Autodesk Inventor part; units mm, degrees
ref_plane "YZ Plane" through (0, 0, 0) normal (1, 0, 0) x (0, 1, 0)
ref_plane "XZ Plane" through (0, 0, 0) normal (0, 1, 0) x (-1, 0, 0)
ref_plane "XY Plane" through (0, 0, 0) normal (0, 0, 1) x (1, 0, 0)
sketch "Sketch1" plane through (0, 0, 0) normal (0, 0, 1) x (1, 0, 0)
  line L0 (5, 0) -> (336, 0)
  line L1 (341, 5) -> (341, 96)
  line L2 (336, 101) -> (5, 101)
  line L3 (0, 96) -> (0, 5)
  arc A0 (5, 101) -> (0, 96) centre (5, 96) ccw
  arc A1 (0, 5) -> (5, 0) centre (5, 5) ccw
  arc A2 (341, 96) -> (336, 101) centre (336, 96) ccw
  arc A3 (336, 0) -> (341, 5) centre (336, 5) ccw
  line L4 (5, 101.2) -> (336, 101.2)
  arc A4 (341.2, 96) -> (336, 101.2) centre (336, 96) ccw
  line L5 (341.2, 96) -> (341.2, 5)
  arc A5 (336, -0.2) -> (341.2, 5) centre (336, 5) ccw
  line L6 (336, -0.2) -> (5, -0.2)
  arc A6 (-0.2, 5) -> (5, -0.2) centre (5, 5) ccw
  line L7 (-0.2, 5) -> (-0.2, 96)
  arc A7 (5, 101.2) -> (-0.2, 96) centre (5, 96) ccw
  line L8 (5, 104) -> (336, 104)
  arc A8 (344, 96) -> (336, 104) centre (336, 96) ccw
  line L9 (344, 96) -> (344, 5)
  arc A9 (336, -3) -> (344, 5) centre (336, 5) ccw
  line L10 (336, -3) -> (5, -3)
  arc A10 (-3, 5) -> (5, -3) centre (5, 5) ccw
  line L11 (-3, 5) -> (-3, 96)
  arc A11 (5, 104) -> (-3, 96) centre (5, 96) ccw
  point P0 (0, 0)
  point P1 (341, 101)
  point P2 (0, 101)
  dimension "d0" = 341
  dimension "d1" = 101
  dimension "d2" = 5
  dimension "d3" = 0.2
  dimension "d4" = 3
extrude "Extrusion1" add sketch "Sketch1" along normal blind 2 contours A1 L3 A0 L2 A2 L1 A3 L0 | L4 A4 L5 A5 L6 A6 L7 A7 | L8 A8 L9 A9 L10 A10 L11 A11
sketch "Sketch2" plane through (0, 0, 2) normal (0, 0, 1) x (1, 0, 0)
  line L0 (5, 104) -> (336, 104)
  line L1 (344, 96) -> (344, 5)
  line L2 (336, -3) -> (5, -3)
  line L3 (-3, 5) -> (-3, 96)
  line L4 (344, 5) -> (344, 96)
  line L5 (5, -3) -> (336, -3)
  arc A0 (5, 104) -> (-3, 96) centre (5, 96) ccw
  arc A1 (-3, 5) -> (5, -3) centre (5, 5) ccw
  arc A2 (336, -3) -> (344, 5) centre (336, 5) ccw
  arc A3 (344, 96) -> (336, 104) centre (336, 96) ccw
  line L6 (336, 101.2) -> (5, 101.2)
  arc A4 (5, 101.2) -> (-0.2, 96) centre (5, 96) ccw
  line L7 (-0.2, 96) -> (-0.2, 5)
  arc A5 (-0.2, 5) -> (5, -0.2) centre (5, 5) ccw
  line L8 (5, -0.2) -> (336, -0.2)
  arc A6 (336, -0.2) -> (341.2, 5) centre (336, 5) ccw
  line L9 (341.2, 5) -> (341.2, 96)
  arc A7 (341.2, 96) -> (336, 101.2) centre (336, 96) ccw
  circle A8 centre (5, 96) radius 2.5
  line L10 (9, 92) -> (332, 92)
  line L11 (332, 92) -> (332, 9)
  line L12 (332, 9) -> (9, 9)
  line L13 (9, 9) -> (9, 92)
  line L14 (-0.2, 89.2) -> (8, 89.2)
  line L15 (8, 89.2) -> (8, 93)
  line L16 (8, 93) -> (11.8, 93)
  line L17 (11.8, 93) -> (11.8, 101.2)
  line L18 (9, 9) -> (332, 92)
  line L19 (170.5, 64.427) -> (170.5, 38.8649)
  line L20 (118.7328, 50.5) -> (212.1169, 50.5)
  circle A9 centre (336, 96) radius 2.5
  line L21 (341.2, 89.2) -> (333, 89.2)
  line L22 (333, 89.2) -> (333, 93)
  line L23 (333, 93) -> (329.2, 93)
  line L24 (329.2, 93) -> (329.2, 101.2)
  circle A10 centre (5, 5) radius 2.5
  line L25 (-0.2, 11.8) -> (8, 11.8)
  line L26 (8, 11.8) -> (8, 8)
  line L27 (8, 8) -> (11.8, 8)
  line L28 (11.8, 8) -> (11.8, -0.2)
  line L29 (329.2, 8) -> (329.2, -0.2)
  line L30 (333, 8) -> (329.2, 8)
  line L31 (333, 11.8) -> (333, 8)
  line L32 (341.2, 11.8) -> (333, 11.8)
  circle A11 centre (336, 5) radius 2.5
  point P0 (0, 0)
  dimension "d7" = 0
  dimension "d8" = 0
  dimension "d9" = 8
  dimension "d10" = 2.8
  dimension "d11" = 5
  dimension "d12" = 5.2
  dimension "d13" = 5.2
  dimension "d19" = 9.2
  dimension "d20" = 9.2
  dimension "d21" = 9.2
  dimension "d22" = 9.2
  dimension "d23" = 1
  dimension "d24" = 1
  dimension "d25" = 12
  dimension "d26" = 12
extrude "Extrusion2" add sketch "Sketch2" along normal blind 30 contours L0 A3 L1 A2 L2 A1 L3 A0 | A7 L9 L21 L22 L23 L24 L6 | L17 L16 L15 L14 L7 A4 L6 | L9 A6 L8 L29 L30 L31 L32 | L25 L26 L27 L28 L8 A5 L7
sketch "Sketch3" plane through (0, 0, 32) normal (0, 0, 1) x (1, 0, 0)
  line L0 (5, 104) -> (336, 104)
  line L1 (344, 96) -> (344, 5)
  line L2 (336, -3) -> (5, -3)
  line L3 (-3, 5) -> (-3, 96)
  arc A0 (5, 104) -> (-3, 96) centre (5, 96) ccw
  arc A1 (-3, 5) -> (5, -3) centre (5, 5) ccw
  arc A2 (336, -3) -> (344, 5) centre (336, 5) ccw
  arc A3 (344, 96) -> (336, 104) centre (336, 96) ccw
  line L4 (336, 101.2) -> (5, 101.2)
  arc A4 (5, 101.2) -> (-0.2, 96) centre (5, 96) ccw
  line L5 (-0.2, 96) -> (-0.2, 5)
  arc A5 (-0.2, 5) -> (5, -0.2) centre (5, 5) ccw
  line L6 (5, -0.2) -> (336, -0.2)
  arc A6 (336, -0.2) -> (341.2, 5) centre (336, 5) ccw
  line L7 (341.2, 5) -> (341.2, 96)
  arc A7 (341.2, 96) -> (336, 101.2) centre (336, 96) ccw
  point P0 (0, 0)
  dimension "d29" = 8
  dimension "d30" = 2.8
extrude "Extrusion3" add sketch "Sketch3" along normal blind 7
sketch "Sketch4" plane through (0, 0, 2) normal (0, 0, 1) x (1, 0, 0)
  line L0 (336, -0.2) -> (5, -0.2)
  line L1 (157.75, -0.2) -> (183.25, -0.2)
  line L2 (183.25, -0.2) -> (183.25, 48.2)
  line L3 (183.25, 48.2) -> (157.75, 48.2)
  line L4 (157.75, 48.2) -> (157.75, -0.2)
  line L5 (-0.2, 5) -> (-0.2, 96)
  circle A0 centre (160.25, 45.7) radius 2.3
  circle A1 centre (180.75, 45.7) radius 2.3
  circle A2 centre (160.25, 2.3) radius 2.3
  circle A3 centre (180.75, 2.3) radius 2.3
  point P0 (0, 0)
  dimension "d33" = 25.5
  dimension "d34" = 48.4
  dimension "d35" = 157.95
  dimension "d36" = 4.6
  dimension "d37" = 4.6
  dimension "d38" = 4.6
  dimension "d39" = 4.6
  dimension "d40" = 2.5
  dimension "d41" = 2.5
  dimension "d42" = 2.5
  dimension "d43" = 2.5
  dimension "d44" = 2.5
  dimension "d45" = 2.5
  dimension "d46" = 2.5
  dimension "d47" = 2.5
extrude "Extrusion4" add sketch "Sketch4" along normal blind 4 contours A0 | A1 | A2 | A3
sketch "Sketch5" plane through (160.25, 2.3, 6) normal (0, 0, 1) x (1, 0, 0)
  circle A0 centre (0, 43.4) radius 2.3
  circle A1 centre (0, 43.4) radius 1.5
  circle A2 centre (20.5, 43.4) radius 2.3
  circle A3 centre (20.5, 43.4) radius 1.5
  circle A4 centre (0, 0) radius 2.3
  circle A5 centre (0, 0) radius 1.5
  circle A6 centre (20.5, 0) radius 2.3
  circle A7 centre (20.5, 0) radius 1.5
  point P0 (-160.25, -2.3)
  dimension "d50" = 3
  dimension "d51" = 3
  dimension "d52" = 3
  dimension "d53" = 3
extrude "Extrusion5" add sketch "Sketch5" along normal blind 3 contours A1 | A3
chamfer "Chamfer1" distance 1 angle 45 2 edges at (158.75, 45.7, 9) (179.25, 45.7, 9)
sketch "Sketch6" plane through (5, -3, 0) normal (0, -1, 0) x (1, 0, 0)
  line L0 (161.3, 2.8) -> (169.7, 2.8)
  line L1 (169.7, 2.8) -> (169.7, 6.2)
  line L2 (169.7, 6.2) -> (161.3, 6.2)
  line L3 (161.3, 6.2) -> (161.3, 2.8)
  line L4 (6.8, 2) -> (324.2, 2)
  line L5 (0, 0) -> (0, 39)
  point P0 (-5, 0)
  dimension "d59" = 8.4
  dimension "d60" = 3.4
  dimension "d61" = 4.2
  dimension "d62" = 161.3
extrude "Extrusion6" cut sketch "Sketch6" against normal blind 3
sketch "Sketch7" plane through (0, 0, 2) normal (0, 0, 1) x (1, 0, 0)
  line L0 (99.8, 7.8) -> (107.8, 7.8)
  line L1 (107.8, 7.8) -> (107.8, 10.8)
  line L2 (107.8, 10.8) -> (99.8, 10.8)
  line L3 (99.8, 10.8) -> (99.8, 7.8)
  line L4 (336, -0.2) -> (5, -0.2)
  line L5 (-0.2, 5) -> (-0.2, 96)
  point P0 (0, 0)
  dimension "d65" = 8
  dimension "d66" = 3
  dimension "d67" = 8
  dimension "d68" = 100
extrude "Extrusion7" cut sketch "Sketch7" against normal blind 3
sketch "Sketch8" plane through (0, 0, 2) normal (0, 0, 1) x (1, 0, 0)
  line L0 (11.8, -0.2) -> (329.2, -0.2)
  line L1 (95.8, -0.2) -> (111.8, -0.2)
  line L2 (111.8, -0.2) -> (111.8, 5.95)
  line L3 (111.8, 5.95) -> (95.8, 5.95)
  line L4 (95.8, 5.95) -> (95.8, -0.2)
  line L5 (107.8, 7.8) -> (99.8, 7.8)
  line L6 (99.8, 7.8) -> (99.8, 10.8)
  point P0 (0, 0)
  dimension "d71" = 16
  dimension "d72" = 1.85
  dimension "d73" = 4
extrude "Extrusion8" add sketch "Sketch8" along normal blind 9
sketch "Sketch9" plane through (0, 0, 39) normal (0, 0, 1) x (1, 0, 0)
  line L0 (-3, -16.474) -> (197, -16.474)
  line L1 (197, -16.474) -> (197, 116.8419)
  line L2 (197, 116.8419) -> (-3, 116.8419)
  line L3 (-3, 116.8419) -> (-3, -16.474)
  line L4 (-3, 96) -> (-3, 5)
  line L5 (197, 116.8419) -> (375.2281, 116.8419)
  line L6 (375.2281, 116.8419) -> (375.2281, -16.474)
  line L7 (375.2281, -16.474) -> (197, -16.474)
  line L8 (197, -16.474) -> (197, 116.8419)
  point P0 (0, 0)
  dimension "d76" = 200
  dimension "d77" = 0
extrude "Extrusion9" cut sketch "Sketch9" against normal blind 50 contours L1 L5 L6 L7
properties part number "Case Left Half"
CAD build for the part. Positions are in the model's coordinates, mm. A direction names the side the tool comes from. Give positions to 0.01 mm unless a question says otherwise; leave off trailing zeros. Write each loop counter-clockwise with the first axis right and the second up, starting at its lowest first coordinate (ties: lowest second). Pieces come first, ordered by that corner, then holes. Notation, with made-up numbers: M 81.5,-12.75 L 118.5,-12.75 A18 ccw 118.5,1.25 Z; hole C 27,43.25 d11. An arc over 180 degrees is marked long. Return JSON: item names as keys, results as strings. Group by question number.
(1) Drill centre lines: L1, parallel to Y at x = 5, z = 13; L2, parallel to Y at x = 87.5, z = 7.5; L3, parallel to Z at x = 9, y = 94. Where is each one in solid material? Low to high. Write a range as [from, to].
(2) 3-axis set-ups, long thin cutter, end or side, ignore diameter. For faces 4 (the face through (-0.719, 101.594, 19.227)), 5 (the face through (7, 7, 32)), 6 (the face through (160, 44, 6)): which of +Z, -Z, +X, -X, +Y, -Y reach the whole face in a straight line?
(3) Mould opens along X. For faces 1 (the face through (4, 89.2, 17)), 2 (the face through (157.952, 2.199, 3.972)), 3 (the face through (1.364, 1.283, 35.451)) say: pulls with the +X half, pulls with the -X half, needs draft (parallel to the pull), parting line crosses it, or undercut.
(4) Band-saw the part on A-A (x = 15). Give the cut face in (y, z).
(5) Flat gauge pins, fed straight in: pin 1 Ø4 at (y, z) = (97, 22.5) entering from +X; pin 2 Ø1.8 at (y, z) = (3, 5) entering from -X; pin 3 Ø4 at (x, y) = (94, 89.5) entering from +Z. Where does each tip first touch, or does it go through?
(6) Band-saw the part on B-B (z = 26.5). Give the cut face in (x, y).
(7) Band-saw the part on C-C (y = 33). Give the cut face in (x, z), and give its area (3 significant figures).
Entries:
{
 "1": {"L1": "y = [-3, 2.5], [7.5, 11.8], [89.2, 93.5], [98.5, 104]", "L2": "y = [-3, -0.2], [101.2, 104]", "L3": "z = [0, 32]"},
 "2": {"face 4": "+Z, -Z, -X, +Y", "face 5": "+Z, +X", "face 6": "+Z"},
 "3": {"face 1": "needs draft", "face 2": "undercut", "face 3": "pulls with the +X half"},
 "4": {"outline": "M -3,0 L 104,0 L 104,39 L 101.2,39 L 101.2,2 L -0.2,2 L -0.2,39 L -3,39 Z"},
 "5": {"pin 1": "stops at x = 11.8", "pin 2": "stops at x = -2.92", "pin 3": "stops at z = 2"},
 "6": {"outline": "M -3,5 A8 ccw 5,-3 L 197,-3 L 197,-0.2 L 11.8,-0.2 L 11.8,8 L 8,8 L 8,11.8 L -0.2,11.8 L -0.2,89.2 L 8,89.2 L 8,93 L 11.8,93 L 11.8,101.2 L 197,101.2 L 197,104 L 5,104 A8 ccw -3,96 Z; hole C 5,5 d5; hole C 5,96 d5"},
 "7": {"outline": "M -3,0 L 197,0 L 197,2 L -0.2,2 L -0.2,39 L -3,39 Z", "area": "504 mm^2"}
}
